from build123d import *

# Parameters (mm, degrees)
ESQUISSE1_W             = 18
ESQUISSE1_H             = 28
BOSS_EXTRU_1_DEPTH      = 10
ESQUISSE3_R             = 4.25
BOSS_EXTRU_2_DEPTH      = 3.5
ESQUISSE4_R             = 1.6
ENL_V_MAT_EXTRU_1_DEPTH = 10.2
ESQUISSE5_R             = 1.6
ENL_V_MAT_EXTRU_2_DEPTH = 10.2
ESQUISSE6_W             = 6.88236931
ESQUISSE6_H             = 23.48997152
BOSS_EXTRU_3_DEPTH      = 1


with BuildPart() as part:
    # Esquisse1 → Boss.-Extru.1 (new body)
    with BuildSketch(Plane.XY):
        with Locations((9, 14)):
            Rectangle(ESQUISSE1_W, ESQUISSE1_H)
    extrude(amount=BOSS_EXTRU_1_DEPTH)

    # Esquisse3 → Boss.-Extru.2 (add)
    with BuildSketch(Plane.XZ):
        with Locations(Location((8.6, 5, 0), (0, 0, 90))):
            Circle(ESQUISSE3_R)
    extrude(amount=BOSS_EXTRU_2_DEPTH)

    # Esquisse4 → Enlèv. mat.-Extru.1 (cut)
    with BuildSketch(Plane(origin=(0, 0, 0), x_dir=(-1, 0, 0), z_dir=(0, 0, -1))):
        with Locations((-15.4, 25.5)):
            Circle(ESQUISSE4_R)
    extrude(amount=-ENL_V_MAT_EXTRU_1_DEPTH, mode=Mode.SUBTRACT)

    # Esquisse5 → Enlèv. mat.-Extru.2 (cut)
    with BuildSketch(Plane(origin=(0, 0, 0), x_dir=(-1, 0, 0), z_dir=(0, 0, -1))):
        with Locations((-15.4, 2.5)):
            Circle(ESQUISSE5_R)
    extrude(amount=-ENL_V_MAT_EXTRU_2_DEPTH, mode=Mode.SUBTRACT)

    # Esquisse6 → Boss.-Extru.3 (add)
    with BuildSketch(Plane.ZY):
        with Locations((5.178101781, 13.870853196)):
            Rectangle(ESQUISSE6_W, ESQUISSE6_H)
    extrude(amount=BOSS_EXTRU_3_DEPTH)


solid = part.part
Design review of the part built by this model. Coordinates are the model's own, in mm. A direction names the side the tool comes from. Coordinates: 2 decimals unless noted, no trailing zeros. Write each loop counter-clockwise with the first axis right and the second up, starting at its lowest first coordinate (ties: lowest second). Pieces come first, ordered by that corner, then holes. Notation, with made-up numbers: (-18, -6.5) - (30, -6.5) arc R23 cw to (30, 8.5) - close; hole circle Ø3 at (35, 19.5). An arc over 180 degrees is marked (long way). One line per item, written item: value.
1) Add section A-A (z = 5). State the section outline as (x, y) points, plus the area to 3 significant figures.
Answer sheet:
outline: (-1, 2.13) - (0, 2.13) - (0, 0) - (4.35, 0) - (4.35, -3.5) - (12.85, -3.5) - (12.85, 0) - (18, 0) - (18, 28) - (0, 28) - (0, 25.62) - (-1, 25.62) - close; hole circle Ø3.2 at (15.4, 2.5); hole circle Ø3.2 at (15.4, 25.5)
area: 541 mm2
2) Mouldability with a two-part tool opening along Y and no side actions: class faces 1 (the face through (4.386, -1.726, 4.447)), 2 (the face through (13.874, 2.981, 4.93)), 3 (the face through (-0.5, 25.616, 5.1)), 4 (the face through (-0.5, 2.126, 5.1)) as +Y half, -Y half, draft (parallel to the pull), parting line (faces both ways), or undercut.
Answer sheet:
face 1: draft
face 2: undercut
face 3: +Y half
face 4: -Y half
3) Add section B-B (y = 2.5). State the section outline as (x, z) points.
Answer sheet:
outline: (-1, 1.74) - (0, 1.74) - (0, 0) - (13.8, 0) - (13.8, 10) - (0, 10) - (0, 8.62) - (-1, 8.62) - close; (17, 0) - (18, 0) - (18, 10) - (17, 10) - close
4) For faces 5 (the face through (-0.5, 13.7, 1.737)), 6 (the face through (-0.5, 13.7, 8.619)), 7 (the face through (9, -3.5, 5)), list the 3-axis set-ups (+Z, -Z, +X, -X, +Y, -Y) from which the entire face can be reached by the end or side of a thin tool; tool diameter is ignored.
Answer sheet:
face 5: -Z, -X, +Y, -Y
face 6: +Z, -X, +Y, -Y
face 7: +Z, -Z, +X, -X, -Y
5) Insertion check: pin 1 (0.5 mm diameter, centred on x = -0.5, y = 15.5, fed in from -Z); pin 2 (0.8 mm diameter, centred on x = -0.5, z = 6, fed in from +Y). Each pin has a flat end and moves straight along its axis. Give the tip position at first contact, or say it passes through.
Answer sheet:
pin 1: stops at z = 1.74
pin 2: stops at y = 25.62
6) To check wall thickness, follow probe 1 along Y at (x, z) = (15.4, 7); probe 2 along Y at (x, z) = (14.25, 2.25); probe 3 along X at (y, z) = (10, 9.25). State the ranges of each line that lie inside material, in increasing order.
Answer sheet:
probe 1: y = 0 to 0.9, 4.1 to 23.9, 27.1 to 28
probe 2: y = 0 to 1.39, 3.61 to 24.39, 26.61 to 28
probe 3: x = 0 to 18
7) Add section C-C (x = 15.4). State the section outline as (y, z) points, plus the area to 3 significant figures.
Answer sheet:
outline: (0, 0) - (0.9, 0) - (0.9, 10) - (0, 10) - close; (4.1, 0) - (23.9, 0) - (23.9, 10) - (4.1, 10) - close; (27.1, 0) - (28, 0) - (28, 10) - (27.1, 10) - close
area: 216 mm2
8) Add section D-D (y = 10.5). State the section outline as (x, z) points.
Answer sheet:
outline: (-1, 1.74) - (0, 1.74) - (0, 0) - (18, 0) - (18, 10) - (0, 10) - (0, 8.62) - (-1, 8.62) - close
